Build history of the part. All positions in model axes, mm. Face numbers are marked on the shaded views. A direction names the side the tool comes from. Give positions to 0.01 mm unless a question says otherwise; leave off trailing zeros. Write each loop counter-clockwise with the first axis right and the second up, starting at its lowest first coordinate (ties: lowest second). Pieces come first, ordered by that corner, then holes. Notation, with made-up numbers: M 14.25,72.25 L 54.25,72.25 A8 cw 54.25,81.25 Z; hole C 9,-10.5 d11. An arc over 180 degrees is marked long. Return JSON: item names as keys, results as strings. Group by question number.
Q1. Tool access for the marked faces 1, 2, 3, 4 and 5: list every direction of +Z, -Z, +X, -X, +Y, -Y with a clear straight run to the whole face (end or side of a thin tool).
Q2. Wall check: probe 1 along X at (y, z) = (-0.25, -4.75); probe 2 along X at (y, z) = (-5.5, 1); probe 3 along Y at (x, z) = (35, 0.25). Give the ranges that are in metal, low to high.
Q3. Flat gauge pins, fed straight in: pin 1 Ø5 at (y, z) = (-0.5, 2) entering from -X; pin 2 Ø1.5 at (x, y) = (36, 2) entering from +Z; pin 3 Ø4 at (x, y) = (25, -2.5) entering from -Z; pin 4 Ø5 at (x, z) = (37.5, -1.5) entering from +Y. Where does each tip first touch, or does it go through?
Q4. Band-saw the part on C-C, the plane y = -4. Give the cut face in (x, z), then the cut area to 3 significant figures.
Q5. Band-saw the part on B-B, the plane x = 36. Give the cut face in (y, z).
Q6. Band-saw the part on A-A, the plane y = 4.25. Give the cut face in (x, z).
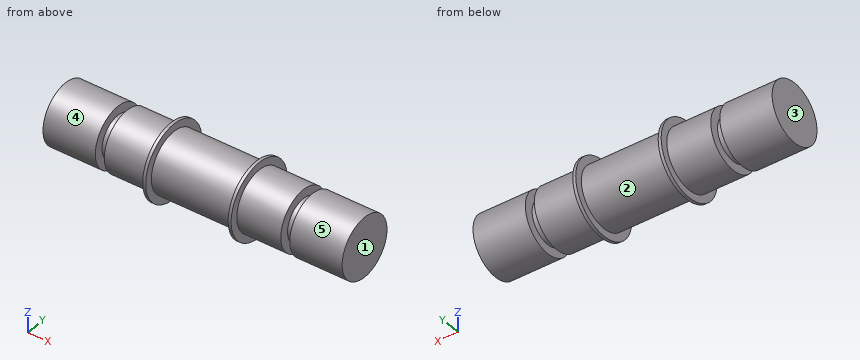
from build123d import *

# Parameters (mm, degrees)
F5_R     = 6.35
F6_DEPTH = 0.508
F7_R     = 6.35
F8_DEPTH = 0.508


with BuildPart() as f1:
    # F0 (on Front) → F1 (revolve)
    with BuildSketch(Plane.XZ):
        Polygon((0, 5.08), (0, 0), (50.8, 0), (50.8, 5.08), (41.91, 5.08), (41.91, 3.556), (40.386, 3.556), (40.386, 5.08), (10.414, 5.08), (10.414, 3.556), (8.89, 3.556), (8.89, 5.08), align=None)
    revolve(axis=Axis((25.4, 0, 0), (-1, 0, 0)))

    # F5 (on offset) → F6 (join)
    with BuildSketch(Plane.YZ.offset(32.4)):
        Circle(F5_R)
    extrude(amount=F6_DEPTH)

    # F7 (on offset) → F8 (join)
    with BuildSketch(Plane.YZ.offset(18.4)):
        Circle(F7_R)
    extrude(amount=-F8_DEPTH)


solid = f1.part
From the geometry:
{
 "1": {"face 1": "+Z, -Z, +X, +Y, -Y", "face 2": "none", "face 3": "+Z, -Z, -X, +Y, -Y", "face 4": "-X", "face 5": "+X"},
 "2": {"probe 1": "x = 0 to 8.89, 10.41 to 40.39, 41.91 to 50.8", "probe 2": "x = 17.89 to 18.4, 32.4 to 32.91", "probe 3": "y = -5.07 to 5.07"},
 "3": {"pin 1": "stops at x = 0", "pin 2": "stops at z = 4.92", "pin 3": "stops at z = -5.06", "pin 4": "stops at y = 5.08"},
 "4": {"outline": "M 0,-3.13 L 8.89,-3.13 L 8.89,3.13 L 0,3.13 Z; M 10.41,-3.13 L 17.89,-3.13 L 17.89,-4.93 L 18.4,-4.93 L 18.4,-3.13 L 32.4,-3.13 L 32.4,-4.93 L 32.91,-4.93 L 32.91,-3.13 L 40.39,-3.13 L 40.39,3.13 L 32.91,3.13 L 32.91,4.93 L 32.4,4.93 L 32.4,3.13 L 18.4,3.13 L 18.4,4.93 L 17.89,4.93 L 17.89,3.13 L 10.41,3.13 Z; M 41.91,-3.13 L 50.8,-3.13 L 50.8,3.13 L 41.91,3.13 Z", "area": "303 mm^2"},
 "5": {"outline": "C 0,0 d10.16"},
 "6": {"outline": "M 0,-2.78 L 8.89,-2.78 L 8.89,2.78 L 0,2.78 Z; M 10.41,-2.78 L 17.89,-2.78 L 17.89,-4.72 L 18.4,-4.72 L 18.4,-2.78 L 32.4,-2.78 L 32.4,-4.72 L 32.91,-4.72 L 32.91,-2.78 L 40.39,-2.78 L 40.39,2.78 L 32.91,2.78 L 32.91,4.72 L 32.4,4.72 L 32.4,2.78 L 18.4,2.78 L 18.4,4.72 L 17.89,4.72 L 17.89,2.78 L 10.41,2.78 Z; M 41.91,-2.78 L 50.8,-2.78 L 50.8,2.78 L 41.91,2.78 Z"}
}
